Check sheet for the modelled part. Datum: model origin and axes. Units: mm. A direction names the side the tool comes from. Coordinates: 2 decimals unless noted, no trailing zeros. Loops run counter-clockwise (first coordinate to the right, second up) from the corner with the lowest first, then second, coordinate; pieces in that order, holes last.
from build123d import *

# Parameters (mm, degrees)
SKETCH1_W                   = 18
SKETCH1_H                   = 18
BOSS_EXTRUDE1_DEPTH         = 35
SKETCH5_W                   = 13
SKETCH5_H                   = 13
CUT_EXTRUDE1_DEPTH          = 30
SKETCH7_W                   = 10.5
SKETCH7_H                   = 20
CUT_EXTRUDE3_DEPTH          = 44.278170017
SKETCH8_W                   = 18
SKETCH8_H                   = 18
BOSS_EXTRUDE2_DEPTH         = 10
SKETCH9_W                   = 11.43
SKETCH9_H                   = 5.85
CUT_EXTRUDE4_DEPTH          = 44.278170017
F_1_4_CLEARANCE_HOLE1_D     = 7.14248
F_1_4_CLEARANCE_HOLE1_DEPTH = 15
F_1_4_CLEARANCE_HOLE1_TIP   = 2.145817477


with BuildPart() as part:
    # Sketch1 → Boss-Extrude1 (new body)
    with BuildSketch(Plane(origin=(0, 0, 0), x_dir=(1, 0, 0), z_dir=(0, 1, 0))):
        with Locations((9, 9)):
            Rectangle(SKETCH1_W, SKETCH1_H)
    extrude(amount=BOSS_EXTRUDE1_DEPTH)

    # Sketch5 → Cut-Extrude1 (cut)
    with BuildSketch(Plane(origin=(0, 35, 0), x_dir=(1, 0, 0), z_dir=(0, 1, 0))):
        with Locations((9, 9)):
            Rectangle(SKETCH5_W, SKETCH5_H)
    extrude(amount=-CUT_EXTRUDE1_DEPTH, mode=Mode.SUBTRACT)

    # Sketch7 → Cut-Extrude3 (cut, through all)
    with BuildSketch(Plane(origin=(18, 0, 0), x_dir=(0, 0, -1), z_dir=(1, 0, 0))):
        with Locations((9.25, 20)):
            Rectangle(SKETCH7_W, SKETCH7_H)
    extrude(amount=-CUT_EXTRUDE3_DEPTH, mode=Mode.SUBTRACT)

    # Sketch8 → Boss-Extrude2 (add)
    with BuildSketch(Plane.XZ):
        with Locations((9, -9)):
            Rectangle(SKETCH8_W, SKETCH8_H)
    extrude(amount=BOSS_EXTRUDE2_DEPTH)

    # Sketch9 → Cut-Extrude4 (cut, through all)
    with BuildSketch(Plane.XY):
        with Locations((9, -2.5)):
            Rectangle(SKETCH9_W, SKETCH9_H)
    extrude(amount=-CUT_EXTRUDE4_DEPTH, mode=Mode.SUBTRACT)

    # 1/4 Clearance Hole1
    with Locations(Plane(origin=(0, -10, 0), x_dir=(-1, 0, 0), z_dir=(0, -1, 0))):
        with Locations((-9, 9)):
            Hole(F_1_4_CLEARANCE_HOLE1_D / 2, depth=F_1_4_CLEARANCE_HOLE1_DEPTH)
            with Locations((0, 0, -(F_1_4_CLEARANCE_HOLE1_DEPTH + F_1_4_CLEARANCE_HOLE1_TIP / 2))):  # 118° drill point
                Cone(0, F_1_4_CLEARANCE_HOLE1_D / 2, F_1_4_CLEARANCE_HOLE1_TIP, mode=Mode.SUBTRACT)


solid = part.part
(1) Section check A-A, the plane y = 12. Enter the section's corners in (x, z), plus the area to 4 significant figures.
(2) Section check D-D, the plane y = 3.5. Enter the section's corners in (x, z), plus the area to 3 significant figures.
(3) Scan lines: line 1 along Z through (x, y) = (9, -6.35); line 2 along Z through (x, y) = (2.75, 13); line 3 along Y through (x, z) = (5.75, -15) (3 decimals). Record each from-to range of solid material in increasing order.
(4) Section check C-C, the plane z = -9. Enter the section's corners in (x, y) (3 decimals).
(5) Draft check along X on faces 5 (the face through (18, 8, -9)), 6 (the face through (17, 35, -9)), 7 (the face through (12, 5, -12)). Enter one of: pulls with the +X half, pulls with the -X half, needs draft (parallel to the pull), parting line crosses it, or undercut.
(6) Section check B-B, the plane x = 14.25. Enter the section's corners in (y, z) (3 decimals), plus the area to 3 significant figures.
(7) Set-up check for faces 1 (the face through (1, 30, -9)), 2 (the face through (14.715, -3, -9)), 3 (the face through (8.226, 2.745, -5.514)), 4 (the face through (2.5, 24, -3)): record each of +Z, -Z, +X, -X, +Y, -Y from which the full face is reachable in a straight line by a thin tool's end or side.
Determined:
1. outline: (0, -18) - (18, -18) - (18, -14.5) - (15.5, -14.5) - (15.5, -15.5) - (2.5, -15.5) - (2.5, -14.5) - (0, -14.5) - close; (0, -4) - (2.5, -4) - (2.5, -2.5) - (15.5, -2.5) - (15.5, -4) - (18, -4) - (18, 0) - (0, 0) - close
1. area: 102.5 mm2
2. outline: (0, -18) - (18, -18) - (18, 0) - (0, 0) - close; hole circle Ø7.14 at (9, -9)
2. area: 284 mm2
3. line 1: z = -18 to -12.57, -5.43 to 0
3. line 2: z = -18 to -15.5, -2.5 to 0
3. line 3: y = -10 to -5.425, 0.425 to 5
4. outline: (0, -10) - (5.429, -10) - (5.429, -5.425) - (3.285, -5.425) - (3.285, 0.425) - (5.429, 0.425) - (5.429, 5) - (2.5, 5) - (2.5, 10) - (0, 10) - close; (0, 30) - (2.5, 30) - (2.5, 35) - (0, 35) - close; (12.571, -10) - (18, -10) - (18, 10) - (15.5, 10) - (15.5, 5) - (12.571, 5) - (12.571, 0.425) - (14.715, 0.425) - (14.715, -5.425) - (12.571, -5.425) - close; (15.5, 30) - (18, 30) - (18, 35) - (15.5, 35) - close
5. face 5: pulls with the +X half
5. face 6: needs draft
5. face 7: undercut
6. outline: (-10, -18) - (-5.425, -18) - (-5.425, 0) - (-10, 0) - close; (0.425, -18) - (35, -18) - (35, -15.5) - (5, -15.5) - (5, -2.5) - (35, -2.5) - (35, 0) - (0.425, 0) - close
6. area: 315 mm2
7. face 1: +X, -X
7. face 2: +Z, -Z
7. face 3: +Y, -Y
7. face 4: +Y
